from build123d import *

# Parameters (mm, degrees)
CROQUIS1_R                 = 1.5
SALIENTE_EXTRUIR1_DEPTH    = 50
CORTAR_EXTRUIR1_DEPTH      = 123.737524824
CORTAR_EXTRUIR1_DEPTH_BACK = 123.737524824
CROQUIS2_W                 = 10.1
CROQUIS2_H                 = 10
CROQUIS2_W_2               = 20.2
REDONDEO3_R                = 3
CROQUIS6_W                 = 80
CROQUIS6_H                 = 15
CORTAR_EXTRUIR5_DEPTH      = 151.214846137
CROQUIS29_W                = 2
CROQUIS29_H                = 60
SALIENTE_EXTRUIR16_DEPTH   = 5
REDONDEO17_R               = 2
CROQUIS19_W                = 60
CROQUIS19_H                = 8
SALIENTE_EXTRUIR10_DEPTH   = 30
REDONDEO12_R               = 15
REDONDEO15_R               = 3
REDONDEO23_R               = 10
CORTAR_EXTRUIR6_DEPTH      = 139.047998899
CORTAR_EXTRUIR4_DEPTH      = 138.71165528
CORTAR_EXTRUIR4_DEPTH_BACK = 138.71165528
CROQUIS4_W                 = 15
CROQUIS4_H                 = 2
REDONDEO24_R               = 3
CROQUIS31_W                = 3
CROQUIS31_H                = 21
CORTAR_EXTRUIR7_DEPTH      = 139.047998899
REDONDEO27_R               = 3


with BuildPart() as part:
    # Croquis1 → Saliente-Extruir1 (new, symmetric)
    with BuildSketch(Plane(origin=(0, 0, 0), x_dir=(0, 0, -1), z_dir=(1, 0, 0))):
        Polygon((-1.5, 11.5), (-1.5, 3.5), (-21.5, 3.5), (-21.5, -11.5), (-111.5, -11.5), (-111.5, 11.5), align=None)
        with Locations((-5, 7.5)):
            Circle(CROQUIS1_R, mode=Mode.SUBTRACT)
    extrude(amount=SALIENTE_EXTRUIR1_DEPTH, both=True)

    # Croquis2 → Cortar-Extruir1 (cut, two sides: drawn at the far end of the back side and taken through both)
    with BuildSketch(Plane(origin=(0, 0, 0), x_dir=(1, 0, 0), z_dir=(0, 1, 0)).offset(-CORTAR_EXTRUIR1_DEPTH_BACK)):
        with Locations((-44.95, -6.5)):
            Rectangle(CROQUIS2_W, CROQUIS2_H)
        with Locations((-25, -6.5)):
            Rectangle(CROQUIS2_W_2, CROQUIS2_H)
        with Locations((0, -6.5)):
            Rectangle(CROQUIS2_W_2, CROQUIS2_H)
        with Locations((25, -6.5)):
            Rectangle(CROQUIS2_W_2, CROQUIS2_H)
        with Locations((44.95, -6.5)):
            Rectangle(CROQUIS2_W, CROQUIS2_H)
    extrude(amount=CORTAR_EXTRUIR1_DEPTH + CORTAR_EXTRUIR1_DEPTH_BACK, mode=Mode.SUBTRACT)

    # Redondeo3
    redondeo3_edges = [part.edges().sort_by_distance(p)[0] for p in [
        (0, 3.5, 21.5),
        (37.5, 11.5, 1.5),
        (12.5, 11.5, 1.5),
        (-12.5, 11.5, 1.5),
        (-37.5, 11.5, 1.5),
        (37.5, 3.5, 1.5),
        (12.5, 3.5, 1.5),
        (-12.5, 3.5, 1.5),
        (-37.5, 3.5, 1.5),
        (-50, 7.5, 11.5),
        (50, 7.5, 11.5),
    ]]
    fillet(redondeo3_edges, radius=REDONDEO3_R)

    # Croquis6 → Cortar-Extruir5 (cut, through all)
    with BuildSketch(Plane.ZY.offset(50)):
        with Locations((71.5, 4)):
            Rectangle(CROQUIS6_W, CROQUIS6_H)
    extrude(amount=-CORTAR_EXTRUIR5_DEPTH, mode=Mode.SUBTRACT)

    # Croquis29 → Saliente-Extruir16 (add)
    with BuildSketch(Plane(origin=(0, -3.5, 0), x_dir=(1, 0, 0), z_dir=(0, 1, 0))):
        with Locations((-46, -61.5)):
            Rectangle(CROQUIS29_W, CROQUIS29_H)
        with Locations((-29, -61.5)):
            Rectangle(CROQUIS29_W, CROQUIS29_H)
        with Locations((-21, -61.5)):
            Rectangle(CROQUIS29_W, CROQUIS29_H)
        with Locations((-4, -61.5)):
            Rectangle(CROQUIS29_W, CROQUIS29_H)
        with Locations((4, -61.5)):
            Rectangle(CROQUIS29_W, CROQUIS29_H)
        with Locations((21, -61.5)):
            Rectangle(CROQUIS29_W, CROQUIS29_H)
        with Locations((29, -61.5)):
            Rectangle(CROQUIS29_W, CROQUIS29_H)
        with Locations((46, -61.5)):
            Rectangle(CROQUIS29_W, CROQUIS29_H)
    extrude(amount=SALIENTE_EXTRUIR16_DEPTH)

    # Redondeo17
    redondeo17_edges = [part.edges().sort_by_distance(p)[0] for p in [
        (-46, -3.5, 91.5),
        (-47, -3.5, 61.5),
        (-46, 1.5, 31.5),
        (-29, -3.5, 91.5),
        (-28, -3.5, 61.5),
        (-29, 1.5, 31.5),
        (-21, -3.5, 91.5),
        (-22, -3.5, 61.5),
        (-21, 1.5, 31.5),
        (-4, -3.5, 91.5),
        (-3, -3.5, 61.5),
        (-4, 1.5, 31.5),
        (4, -3.5, 91.5),
        (3, -3.5, 61.5),
        (4, 1.5, 31.5),
        (21, -3.5, 91.5),
        (22, -3.5, 61.5),
        (21, 1.5, 31.5),
        (29, -3.5, 91.5),
        (28, -3.5, 61.5),
        (29, 1.5, 31.5),
        (46, -3.5, 91.5),
        (47, -3.5, 61.5),
        (46, 1.5, 31.5),
    ]]
    fillet(redondeo17_edges, radius=REDONDEO17_R)

    # Croquis19 → Saliente-Extruir10 (add)
    with BuildSketch(Plane.ZY.offset(50)):
        with Locations((81.5, -7.5)):
            Rectangle(CROQUIS19_W, CROQUIS19_H)
    extrude(amount=SALIENTE_EXTRUIR10_DEPTH)

    # Redondeo12
    redondeo12_edges = [part.edges().sort_by_distance(p)[0] for p in [
        (50, -7.5, 111.5),
    ]]
    fillet(redondeo12_edges, radius=REDONDEO12_R)

    # Redondeo15
    redondeo15_edges = [part.edges().sort_by_distance(p)[0] for p in [
        (0, 11.5, 31.5),
    ]]
    fillet(redondeo15_edges, radius=REDONDEO15_R)

    # Redondeo23
    redondeo23_edges = [part.edges().sort_by_distance(p)[0] for p in [
        (-50, -7.5, 51.5),
    ]]
    fillet(redondeo23_edges, radius=REDONDEO23_R)

    # Croquis30 → Cortar-Extruir6 (cut, through all)
    with BuildSketch(Plane(origin=(0, -3.5, 0), x_dir=(1, 0, 0), z_dir=(0, 1, 0))):
        with BuildLine():
            Line((-80, -64), (-74.341640786, -61.170820393))
            ThreePointArc((-74.341640786, -61.170820393), (-71.422806664, -61.302149541), (-70, -63.854101966))
            Line((-70, -63.854101966), (-70, -99.145898034))
            ThreePointArc((-70, -99.145898034), (-71.422806664, -101.697850459), (-74.341640786, -101.829179607))
            Line((-74.341640786, -101.829179607), (-80, -99))
            Line((-80, -99), (-80, -64))
        make_face()
    extrude(amount=-CORTAR_EXTRUIR6_DEPTH, mode=Mode.SUBTRACT)

    # Croquis4 → Cortar-Extruir4 (cut, two sides: drawn at the far end of the back side and taken through both)
    with BuildSketch(Plane(origin=(0, 0, 0), x_dir=(0, 0, -1), z_dir=(1, 0, 0)).offset(-CORTAR_EXTRUIR4_DEPTH_BACK)):
        with Locations((-86.5, -8.5)):
            Rectangle(CROQUIS4_W, CROQUIS4_H)
        with Locations((-31.5, -8.5)):
            Rectangle(CROQUIS4_W, CROQUIS4_H)
    extrude(amount=CORTAR_EXTRUIR4_DEPTH + CORTAR_EXTRUIR4_DEPTH_BACK, mode=Mode.SUBTRACT)

    # Redondeo24
    redondeo24_edges = [part.edges().sort_by_distance(p)[0] for p in [
        (-80, -7.5, 111.5),
        (-80, -7.5, 51.5),
    ]]
    fillet(redondeo24_edges, radius=REDONDEO24_R)

    # Croquis31 → Cortar-Extruir7 (cut, through all)
    with BuildSketch(Plane(origin=(0, -3.5, 0), x_dir=(1, 0, 0), z_dir=(0, 1, 0))):
        with Locations((-68.5, -86.5)):
            Rectangle(CROQUIS31_W, CROQUIS31_H)
    extrude(amount=-CORTAR_EXTRUIR7_DEPTH, mode=Mode.SUBTRACT)

    # Redondeo27
    redondeo27_edges = [part.edges().sort_by_distance(p)[0] for p in [
        (-67, -7.5, 76),
        (-67, -7.5, 97),
    ]]
    fillet(redondeo27_edges, radius=REDONDEO27_R - 0.0001)  # a hair under: the kernel refuses the full size


solid = part.part
Could you check a few things on this model? Use its own coordinates, in mm. A direction names the side the tool comes from. Round coordinates to 2 decimals unless told otherwise and drop trailing zeros. Order: outer loops, then holes, each group sorted by start corner. A loop starts at its lowest first (then second) coordinate and runs counter-clockwise, first axis right, second up.
Q1. Thinking about a two-plate mould opening in Z: for faces 1 (the face through (45.49, -7.44, 107.22)), 2 (the face through (14.9, 7, 7)), 3 (the face through (-1, -7.5, 32)), which applies, released by +Z, released by -Z, zero draft, split by the parting line, or undercut?
Geometry says:
face 1: released by +Z
face 2: zero draft
face 3: undercut
Q2. I'm going to push flat-ended pins straight in: P1, Ø5, axis at x = -64.5, y = -5.5, coming from the -Z side; P2, Ø11, axis at x = -12, z = 11, coming from the -Y side; P3, Ø2, axis at x = 21, y = 0.5, coming from the +Z side; P4, Ø2.5, axis at y = 7.5, z = 5, coming from the -X side. Where does each tip first touch, or does it pass through?
Geometry says:
P1: stops at z = 51.5
P2: stops at y = 3.5
P3: stops at z = 91.5
P4: passes through
Q3. Which directions (+Z, -Z, +X, -X, +Y, -Y) give clear straight access to the entire face, cutting with the end or side of a thin tool? Please do faces 4 (the face through (-30, -2, 63)), 5 (the face through (-71.387, -7.444, 101.675)), 6 (the face through (1, 3.5, 15)), 7 (the face through (-35.1, 7, 7)).
Geometry says:
face 4: +Z, +Y
face 5: +Y, -Y
face 6: -Z, +X, -X, -Y
face 7: -Z, +Y, -Y
Q4. Imagine slicing it at A-A, the plane x = -65.5. List the corners of the cut face in (y, z) for me, then the cut area to 3 significant figures.
Geometry says:
outline: (-11.5, 51.5) - (-3.5, 51.5) - (-3.5, 111.5) - (-11.5, 111.5) - close; hole (-9.5, 79) - (-7.5, 79) - (-7.5, 94) - (-9.5, 94) - close
area: 450 mm2
Q5. Please list where these lines run through material, in increasing order: probe 1 along Y at (x, z) = (37, 5); probe 2 along Z at (x, y) = (37, 7.5); probe 3 along Z at (x, y) = (-44.5, -2.75).
Geometry says:
probe 1: y = 3.5 to 6, 9 to 11.5
probe 2: z = 1.5 to 3.5, 6.5 to 31.5
probe 3: z = 21.5 to 31.5
